The model under review builds one solid part; all positions refer to its coordinate system, in mm. Give positions to 0.01 mm unless a question says otherwise; leave off trailing zeros. Order: outer loops, then holes, each group sorted by start corner. A loop starts at its lowest first (then second) coordinate and runs counter-clockwise, first axis right, second up. Notation, with made-up numbers: (57.25, 28.5) - (111.25, 28.5) arc R23 ccw to (111.25, 57.5) - close; hole circle Ø11 at (80, 55). An arc over 180 degrees is marked (long way). Put each result on its own line as item: value.
```python
from build123d import *

# Parameters (mm, degrees)
SKETCH_1_R               = 62
EXTRUDE_1_DEPTH          = 22
SKETCH_3_R               = 9
CHAMFER_3_SIZE           = 2
CHAMFER_2_SIZE           = 2
SKETCH_4_R               = 18
EXTRUDE_2_DEPTH          = 16
CHAMFER_4_SIZE           = 10
FILLET_1_R               = 20
SKETCH_5_R               = 1.8
CUT_EXTRUDE_1_DEPTH      = 96.561498523
SKETCH_6_R               = 4
CUT_EXTRUDE_2_DEPTH      = 22
CHAMFER_5_SIZE           = 2.4
CHAMFER_6_SIZE           = 1
CHAMFER_7_SIZE           = 1
CUT_EXTRUDE_3_DEPTH      = 96.561498523
CUT_EXTRUDE_3_DEPTH_BACK = 96.561498523
SKETCH_7_R               = 2
SKETCH_7_R_2             = 3
CHAMFER_8_SIZE           = 2
CHAMFER_9_SIZE           = 0.5
CHAMFER_10_SIZE          = 1


with BuildPart() as part:
    # Эскиз1 → Бобышка-Вытянуть1 (new body)
    with BuildSketch(Plane(origin=(0, 0, 0), x_dir=(1, 0, 0), z_dir=(0, 1, 0))):
        with Locations(Location((0, 0, 0), (0, 0, 270))):
            Circle(SKETCH_1_R)
    extrude(amount=EXTRUDE_1_DEPTH)

    # Эскиз3 → Вырез-Повернуть2 (revolve, cut)
    with BuildSketch(Plane.XY, mode=Mode.PRIVATE) as cut_revolve_2_sk:
        with Locations((-65, 11)):
            Circle(SKETCH_3_R)
    revolve(cut_revolve_2_sk.sketch.rotate(Axis((0, 0, 0), (0, 1, 0)), 180), axis=Axis((0, 0, 0), (0, 1, 0)), mode=Mode.SUBTRACT)

    # Фаска3
    chamfer_3_edges = [part.edges().sort_by_distance(p)[0] for p in [
        (0, 0, -62),
    ]]
    chamfer(chamfer_3_edges, length=CHAMFER_3_SIZE)

    # Фаска2
    chamfer_2_edges = [part.edges().sort_by_distance(p)[0] for p in [
        (0, 22, -62),
    ]]
    chamfer(chamfer_2_edges, length=CHAMFER_2_SIZE)

    # Эскиз4 → Бобышка-Вытянуть2 (add)
    with BuildSketch(Plane(origin=(0, 22, 0), x_dir=(1, 0, 0), z_dir=(0, 1, 0))):
        with Locations(Location((0, 0, 0), (0, 0, 270))):
            Circle(SKETCH_4_R)
    extrude(amount=EXTRUDE_2_DEPTH)

    # Фаска4
    chamfer_4_edges = [part.edges().sort_by_distance(p)[0] for p in [
        (0, 22, -18),
    ]]
    chamfer(chamfer_4_edges, length=CHAMFER_4_SIZE)

    # Скругление1
    fillet_1_edges = [part.edges().sort_by_distance(p)[0] for p in [
        (0, 22, -28),
    ]]
    fillet(fillet_1_edges, radius=FILLET_1_R)

    # Эскиз5 → Вырез-Вытянуть1 (cut, through all)
    with BuildSketch(Plane(origin=(0, 38, 0), x_dir=(1, 0, 0), z_dir=(0, 1, 0))):
        with Locations(Location((0, 13.5, 0), (0, 0, 270))):
            Circle(SKETCH_5_R)
        with Locations(Location((11.691342951, -6.75, 0), (0, 0, 270))):
            Circle(SKETCH_5_R)
        with Locations(Location((-11.691342951, -6.75, 0), (0, 0, 270))):
            Circle(SKETCH_5_R)
    extrude(amount=-CUT_EXTRUDE_1_DEPTH, mode=Mode.SUBTRACT)

    # Эскиз6 → Вырез-Вытянуть2 (cut)
    with BuildSketch(Plane.XZ):
        with Locations(Location((0, -13.5, 0), (0, 0, 270))):
            Circle(SKETCH_6_R)
        with Locations(Location((11.691342951, 6.75, 0), (0, 0, 270))):
            Circle(SKETCH_6_R)
        with Locations(Location((-11.691342951, 6.75, 0), (0, 0, 270))):
            Circle(SKETCH_6_R)
    extrude(amount=-CUT_EXTRUDE_2_DEPTH, mode=Mode.SUBTRACT)

    # Фаска5
    # the kernel refuses this chamfer: 2.4 mm, written as the material it adds along each edge
    with BuildSketch(Plane(origin=(0, 22, -13.5), x_dir=(0, 0, -1), z_dir=(-1, 0, 0))) as chamfer_5_piece_1_section:
        Polygon((4 - CHAMFER_5_SIZE, 0), (4, CHAMFER_5_SIZE), (4, 0), align=None)
    chamfer_5_piece_1 = revolve(axis=Axis((0, 22, -13.5), (0, -1, 0)), mode=Mode.PRIVATE)
    chamfer_5_piece_1 = chamfer_5_piece_1 - Plane(origin=(0, 20.694254698, -13.5), x_dir=(0, 0, 1), z_dir=(0, 1, 0)) * Cylinder(1.8, 16, mode=Mode.PRIVATE)
    add(chamfer_5_piece_1)
    with BuildSketch(Plane(origin=(-11.691342951, 22, 6.75), x_dir=(0, 0, -1), z_dir=(-1, 0, 0))) as chamfer_5_piece_2_section:
        Polygon((4 - CHAMFER_5_SIZE, 0), (4, CHAMFER_5_SIZE), (4, 0), align=None)
    chamfer_5_piece_2 = revolve(axis=Axis((-11.691342951, 22, 6.75), (0, -1, 0)), mode=Mode.PRIVATE)
    chamfer_5_piece_2 = chamfer_5_piece_2 - Plane(origin=(-11.691342951, 20.694254698, 6.75), x_dir=(0, 0, 1), z_dir=(0, 1, 0)) * Cylinder(1.8, 17, mode=Mode.PRIVATE)
    add(chamfer_5_piece_2)
    with BuildSketch(Plane(origin=(11.691342951, 22, 6.75), x_dir=(0, 0, -1), z_dir=(-1, 0, 0))) as chamfer_5_piece_3_section:
        Polygon((4 - CHAMFER_5_SIZE, 0), (4, CHAMFER_5_SIZE), (4, 0), align=None)
    chamfer_5_piece_3 = revolve(axis=Axis((11.691342951, 22, 6.75), (0, -1, 0)), mode=Mode.PRIVATE)
    chamfer_5_piece_3 = chamfer_5_piece_3 - Plane(origin=(11.691342951, 20.694254698, 6.75), x_dir=(0, 0, 1), z_dir=(0, 1, 0)) * Cylinder(1.8, 17, mode=Mode.PRIVATE)
    add(chamfer_5_piece_3)

    # Фаска6
    chamfer_6_edges = [part.edges().sort_by_distance(p)[0] for p in [
        (0, 0, -9.5),
        (11.691342951, 0, 10.75),
        (-11.691342951, 0, 10.75),
    ]]
    chamfer(chamfer_6_edges, length=CHAMFER_6_SIZE)

    # Фаска7
    chamfer_7_edges = [part.edges().sort_by_distance(p)[0] for p in [
        (0, 38, -18),
    ]]
    chamfer(chamfer_7_edges, length=CHAMFER_7_SIZE)

    # Эскиз7 → Вырез-Вытянуть3 (cut, two sides: drawn at the far end of the back side and taken through both)
    with BuildSketch(Plane(origin=(0, 38, 0), x_dir=(1, 0, 0), z_dir=(0, 1, 0)).offset(-CUT_EXTRUDE_3_DEPTH_BACK)):
        with Locations(Location((0, 50, 0), (0, 0, 270))):
            Circle(SKETCH_7_R)
        with Locations(Location((35.355339059, 35.355339059, 0), (0, 0, 270))):
            Circle(SKETCH_7_R)
        with Locations(Location((50, 0, 0), (0, 0, 270))):
            Circle(SKETCH_7_R)
        with Locations(Location((35.355339059, -35.355339059, 0), (0, 0, 270))):
            Circle(SKETCH_7_R)
        with Locations(Location((0, -50, 0), (0, 0, 270))):
            Circle(SKETCH_7_R)
        with Locations(Location((-35.355339059, -35.355339059, 0), (0, 0, 270))):
            Circle(SKETCH_7_R)
        with Locations(Location((-50, 0, 0), (0, 0, 270))):
            Circle(SKETCH_7_R)
        with Locations(Location((-35.355339059, 35.355339059, 0), (0, 0, 270))):
            Circle(SKETCH_7_R)
        with Locations(Location((0, 0, 0), (0, 0, 270))):
            Circle(SKETCH_7_R_2)
    extrude(amount=CUT_EXTRUDE_3_DEPTH + CUT_EXTRUDE_3_DEPTH_BACK, mode=Mode.SUBTRACT)

    # Фаска8
    chamfer_8_edges = [part.edges().sort_by_distance(p)[0] for p in [
        (-35.355339059, 22, 33.355339059),
        (0, 22, 48),
        (35.355339059, 22, -37.355339059),
        (50, 22, -2),
        (35.355339059, 22, 33.355339059),
        (0, 22, -52),
        (-35.355339059, 22, -37.355339059),
        (-50, 22, -2),
    ]]
    chamfer(chamfer_8_edges, length=CHAMFER_8_SIZE)

    # Фаска9
    chamfer_9_edges = [part.edges().sort_by_distance(p)[0] for p in [
        (0, 38, -3),
        (0, 38, -15.3),
        (11.691342951, 38, 4.95),
        (-11.691342951, 38, 4.95),
    ]]
    chamfer(chamfer_9_edges, length=CHAMFER_9_SIZE)

    # Фаска10
    chamfer_10_edges = [part.edges().sort_by_distance(p)[0] for p in [
        (-35.355339059, 0, 33.355339059),
        (0, 0, 48),
        (0, 0, -3),
        (35.355339059, 0, -37.355339059),
        (50, 0, -2),
        (35.355339059, 0, 33.355339059),
        (0, 0, -52),
        (-35.355339059, 0, -37.355339059),
        (-50, 0, -2),
    ]]
    chamfer(chamfer_10_edges, length=CHAMFER_10_SIZE)


solid = part.part
```
(1) Take a section at C-C, the plane y = 23.5. Write out the cut boundary in (x, z), then the cut area to 3 significant figures.
The answers:
outline: circle Ø57.37 at (0, 0); hole circle Ø3.6 at (-11.69, 6.75); hole circle Ø6 at (0, 0); hole circle Ø3.6 at (0, -13.5); hole circle Ø3.6 at (11.69, 6.75)
area: 2,530 mm^2
(2) The part is to be moulded in two halves that separate along X. For faces 1 (the flat face through (1, 0, 12)), 2 (the cylindrical face through (-37.13, 10.37, 36.28)), 3 (the cylindrical face through (61.472, 2.254, -8.071)), say which applies: pulls with the +X half, pulls with the -X half, needs draft (parallel to the pull), parting line crosses it, or undercut.
The answers:
face 1: needs draft
face 2: undercut
face 3: parting line crosses it
(3) Wall thickness on L1, parallel to Z at x = -0.5, y = 32.5; L2, parallel to Y at x = 14.5, z = 57.5; L3, parallel to X at y = 10.25, z = 6.75: over which ranges is each line inside the solid? List them lowest first.
The answers:
L1: -17.99 to -15.23, -11.77 to -2.96, 2.96 to 17.99
L2: 0 to 4.04, 17.96 to 22
L3: -55.62 to -15.69, -7.69 to 7.69, 15.69 to 55.62
(4) Take a section at A-A, the plane y = 13.5. Count the separate pieces of the cut face and the enclosed holes in it, then the cut area to 3 significant figures.
The answers:
separate pieces: 1
enclosed holes: 12
area: 9,700 mm^2
(5) Clearance check with flat-ended pins moving along their axes: pin 1 Ø2 at (x, z) = (0, -13.5) entering from +Y; pin 2 Ø4.5 at (x, z) = (11.69, 6.75) entering from -Y; pin 3 Ø5 at (x, z) = (35.36, -35.36) entering from -Y; pin 4 Ø7 at (x, z) = (0, -13.5) entering from -Y. State where each tip first meets the part, or that it passes through.
The answers:
pin 1: through
pin 2: y = 21.35
pin 3: y = 0.49
pin 4: y = 20.1
